Autodesk Fusion 360 part; units mm, degrees
sketch "Sketch1" plane through (0, 0, 0) normal (0, 1, 0) x (1, 0, 0)
  line L0 (20, -20) -> (-20, -20)
  line L1 (-20, -20) -> (-20, 20)
  line L2 (-20, 20) -> (20, 20)
  line L3 (20, 20) -> (20, -20)
  line L4 (20, -20) -> (-20, 20) construction
  line L5 (-20, -20) -> (20, 20) construction
  line L6 (-20, 4) -> (-15, 4)
  line L7 (-15, 4) -> (-15, -4)
  line L8 (-15, -4) -> (-20, -4)
  line L9 (-20, -4) -> (-20, 4)
  line L10 (-4, 20) -> (4, 20)
  line L11 (4, 20) -> (4, 15)
  line L12 (4, 15) -> (-4, 15)
  line L13 (-4, 15) -> (-4, 20)
  line L14 (20, 4) -> (15, 4)
  line L15 (15, 4) -> (15, -4)
  line L16 (15, -4) -> (20, -4)
  line L17 (20, -4) -> (20, 4)
  line L18 (-4, -20) -> (4, -20)
  line L19 (4, -20) -> (4, -15)
  line L20 (4, -15) -> (-4, -15)
  line L21 (-4, -15) -> (-4, -20)
  dimension "d1" = 40
  dimension "d2" = 40
  dimension "d3" = 5
  dimension "d4" = 8
  dimension "d5" = 16
  dimension "d6" = 5
  dimension "d7" = 16
  dimension "d8" = 8
  dimension "d9" = 5
  dimension "d10" = 5
  dimension "d11" = 8
  dimension "d12" = 8
  dimension "d13" = 16
  dimension "d14" = 16
extrude "Extrude1" add sketch "Sketch1" against normal blind 3 contours L0 L1 L2 L3 L6 L7 L8 L11 L12 L13 L14 L15 L16 L19 L20 L21
extrude "Extrude2" add sketch "Sketch1" against normal blind 8 contours L0 L18 L19 L20 L21 | L3 L14 L15 L16 L17 | L1 L6 L7 L8 L9 | L2 L10 L11 L12 L13
hole "Hole1" at (0, 0, 0) direction (0, -1, 0) diameter 9 depth 30 tip angle 118
fillet "Fillet1" radius 4 4 edges at (20, -1.5, -20) (-20, -1.5, -20) (20, -1.5, 20) (-20, -1.5, 20)
sketch "Sketch2" plane through (0, 0, 0) normal (0, 1, 0) x (1, 0, 0)
  line L0 (-17.5, 15) -> (17.5, 15)
  line L1 (17.5, 15) -> (17.5, -15)
  line L2 (17.5, -15) -> (-17.5, -15)
  line L3 (-17.5, -15) -> (-17.5, 15)
  dimension "d24" = 35
  dimension "d25" = 30
  dimension "d26" = 15
  dimension "d27" = 17.5
extrude "Extrude3" add sketch "Sketch2" along normal blind 30
sketch "Sketch3" plane through (0, 30, 0) normal (0, 1, 0) x (-1, 0, 0)
  line L0 (17.5, 15) -> (-17.5, 15)
  line L1 (-17.5, 15) -> (-17.5, -15)
  line L2 (-17.5, -15) -> (17.5, -15)
  line L3 (17.5, -15) -> (17.5, 15)
  circle A0 centre (0, 0) radius 4.5
hole "Hole2" at (0, 30, 0) direction (0, -1, 0) diameter 9 depth 90 tip angle 118 counterbore diameter 15 counterbore depth 28
equation "d6 = d3"
equation "d7 = d5"
equation "d8 = d4"
equation "d9 = d3"
equation "d10 = d3"
equation "d11 = d4"
equation "d12 = d4"
equation "d13 = d7"
equation "d14 = d7"
Input: part model. Units: mm. Frame: model coordinates. A direction names the side the tool comes from. Round coordinates to 2 decimals unless told otherwise and drop trailing zeros. Order: outer loops, then holes, each group sorted by start corner. A loop starts at its lowest first (then second) coordinate and runs counter-clockwise, first axis right, second up. Notation, with made-up numbers: (6.25, 22) - (52.25, 22) arc R13 cw to (52.25, 34) - close; hole circle Ø5 at (-39, -16.75). An arc over 180 degrees is marked (long way). Use a Markdown table: item, result.
1. Section C-C on y = 11. Return the cut outline in (x, z), then the cut area to 3 significant figures.
Evaluation:
| item | result |
|---|---|
| outline | (-17.5, -15) - (17.5, -15) - (17.5, 15) - (-17.5, 15) - close; hole circle Ø15 at (0, 0) |
| area | 873 mm^2 |
2. Mould query, pull axis X, two halves, no side actions, for faces 1 (the face through (5, 2, 0)), 2 (the face through (-17.5, 15, 0)), 3 (the face through (0, 15, 15)). Classes: +X half, -X half, draft (parallel to the pull), parting line (faces both ways), or undercut.
Evaluation:
| item | result |
|---|---|
| face 1 | undercut |
| face 2 | -X half |
| face 3 | draft |
3. Material intervals for probe 1 along Z at (x, y) = (-2.5, -4); probe 2 along Z at (x, y) = (0, -0.35), sorted ascending.
Evaluation:
| item | result |
|---|---|
| probe 1 | -20 to -15, 15 to 20 |
| probe 2 | -20 to -4.5, 4.5 to 20 |
4. Section A-A on z = 0. Return the cut outline in (x, y), then the cut area to 3 significant figures.
Evaluation:
| item | result |
|---|---|
| outline | (-20, -8) - (-15, -8) - (-15, -3) - (-4.5, -3) - (-4.5, 2) - (-7.5, 2) - (-7.5, 30) - (-17.5, 30) - (-17.5, 0) - (-20, 0) - close; (4.5, -3) - (15, -3) - (15, -8) - (20, -8) - (20, 0) - (17.5, 0) - (17.5, 30) - (7.5, 30) - (7.5, 2) - (4.5, 2) - close |
| area | 755 mm^2 |
5. Access query for faces 4 (the face through (-0.33, 15.804, -7.493)), 5 (the face through (-15, -5, 0)), 6 (the face through (-18, -5, -4)). Directions: +Z, -Z, +X, -X, +Y, -Y. A direction counts if a zero-diameter tool reaches every point of the face in a straight line with its end or side. Return the directions, or none.
Evaluation:
| item | result |
|---|---|
| face 4 | +Y |
| face 5 | +Z, -Z, -Y |
| face 6 | -Z, +X, -X, -Y |
6. Section D-D on x = -14. Return the cut outline in (y, z).
Evaluation:
| item | result |
|---|---|
| outline | (-3, -20) - (0, -20) - (0, -15) - (30, -15) - (30, 15) - (0, 15) - (0, 20) - (-3, 20) - close |
7. Section B-B on x = 0. Return the cut outline in (y, z).
Evaluation:
| item | result |
|---|---|
| outline | (-8, -20) - (0, -20) - (0, -15) - (30, -15) - (30, -7.5) - (2, -7.5) - (2, -4.5) - (-3, -4.5) - (-3, -15) - (-8, -15) - close; (-8, 15) - (-3, 15) - (-3, 4.5) - (2, 4.5) - (2, 7.5) - (30, 7.5) - (30, 15) - (0, 15) - (0, 20) - (-8, 20) - close |
8. First-contact query: pin 1 (2 mm diameter, centred on x = 1, z = 6.5, fed in from -Y); pin 2 (4 mm diameter, centred on y = 17, z = 8, fed in from +X); pin 3 (9 mm diameter, centred on x = -4.5, y = 20.5, fed in from +Z). Flat tips, straight axial feed; report the tip coordinate or a pass-through.
Evaluation:
| item | result |
|---|---|
| pin 1 | y = -3 |
| pin 2 | x = 17.5 |
| pin 3 | z = 15 |
